CAD build for the part. Positions are in the model's coordinates, mm. A direction names the side the tool comes from. Coordinates: 2 decimals unless noted, no trailing zeros. Write each loop counter-clockwise with the first axis right and the second up, starting at its lowest first coordinate (ties: lowest second). Pieces come first, ordered by that corner, then holes. Notation, with made-up numbers: (27.5, -4.75) - (33.5, -4.75) arc R36 cw to (33.5, 33.25) - close; hole circle Ø2 at (86, -12.5). An arc over 180 degrees is marked (long way). One line per question, with ' | ' between items. Start each with the question number.
1. Band-saw the part on D-D, the plane y = -25. Write the cut outline in (x, z), then the cut area to 3 significant figures.
2. Flat gauge pins, fed straight in: P1, Ø1.5, axis at y = 67, z = 3, coming from the -X side; P2, Ø1, axis at x = 87, y = 21.5, coming from the +Z side. Where does each tip first touch, or does it go through?
3. Band-saw the part on B-B, the plane y = 37. Write the cut outline in (x, z).
4. Probe line 1 (X direction, y = -22, z = 1.15); line 2 (Y direction, x = 71, z = 1.3); line 3 (X direction, y = 14.5, z = 1.85). List the from-to ranges inside material, lowest first.
5. Band-saw the part on C-C, the plane x = 55.5. Write the cut outline in (y, z).
6. Which spindle directions (+Z, -Z, +X, -X, +Y, -Y) get a long thin tool onto all of the face, cutting with end or side? Do faces 1 (the flat face through (113, -11, 2)), 2 (the flat face through (-34.409, 38, 3)), 3 (the flat face through (113, 66.124, 3)), 4 (the flat face through (-29.409, 67, 2)). Say none if no direction does.
7. Band-saw the part on A-A, the plane x = 13. Write the cut outline in (y, z), then the cut area to 3 significant figures.
from build123d import *

# Parameters (mm, degrees)
F0_W     = 160
F0_H     = 110
F1_DEPTH = 2
F2_W     = 155
F2_H     = 5
F3_DEPTH = 3
F4_W     = 0.4
F4_H     = 100.6983700028
F4_H_2   = 0.4
F4_W_2   = 91.7048521668
F4_W_3   = 70
F4_H_3   = 101.3179807599
F4_H_4   = 104.9661831624
F4_H_5   = 97.0501676003
F4_W_4   = 42.9082732886
F5_DEPTH = 0.6
F6_DEPTH = 4
F6_TAPER = -15
F7_R     = 2
F8_W     = 10
F8_H     = 10
F8_W_2   = 47.3290588707
F8_H_2   = 24.0664053708
F8_W_3   = 54.0067385882
F8_H_3   = 33.9830359444
F8_W_4   = 52.8240427375
F8_H_4   = 37.9707552493
F8_W_5   = 50.7075823843
F8_H_5   = 33.7607157417
F9_DEPTH = 25


with BuildPart() as f1:
    # F0 (on Top) → F1 (new body)
    with BuildSketch(Plane.XY):
        with Locations((40.5911064893, 16.1241146261)):
            Rectangle(F0_W, F0_H)
    extrude(amount=F1_DEPTH)

    # F2 (on face) → F3 (join)
    with BuildSketch(Plane.XY.offset(2)):
        Polygon((-34.4088935107, 71.1241146261), (-39.4088935107, 71.1241146261), (-39.4088935107, -38.8758853739), (-34.4088935107, -38.8758853739), (-34.4088935107, 66.1241146261), align=None)
        with Locations((43.0911064893, 68.6241146261)):
            Rectangle(F2_W, F2_H)
    extrude(amount=F3_DEPTH)

    # F4 (on face) → F5 (cut)
    with BuildSketch(Plane.XY.offset(2)):
        with Locations((35.5911064893, 66.6732996275)):
            Rectangle(F4_W, F4_H)
        with Locations((35.5911064893, 16.1241146261)):
            Rectangle(F4_W, F4_H_2)
        with Locations((-10.4613195941, 16.1241146261)):
            Rectangle(F4_W_2, F4_H_2)
        with Locations((70.7911064893, 16.1241146261)):
            Rectangle(F4_W_3, F4_H_2)
        with Locations((35.5911064893, -34.7348757538)):
            Rectangle(F4_W, F4_H_3)
        with Locations((105.9911064893, 16.1241146261)):
            Rectangle(F4_W, F4_H_2)
        with Locations((105.9911064893, 68.8072062073)):
            Rectangle(F4_W, F4_H_4)
        with Locations((105.9911064893, -32.600969174)):
            Rectangle(F4_W, F4_H_5)
        with Locations((127.6452431336, 16.1241146261)):
            Rectangle(F4_W_4, F4_H_2)
    extrude(amount=-F5_DEPTH, mode=Mode.SUBTRACT)

    # F4 (on face) → F6 (cut)
    with BuildSketch(Plane.XY.offset(2)):
        with Locations((35.5911064893, 66.6732996275)):
            Rectangle(F4_W, F4_H)
        with Locations((35.5911064893, 16.1241146261)):
            Rectangle(F4_W, F4_H_2)
        with Locations((-10.4613195941, 16.1241146261)):
            Rectangle(F4_W_2, F4_H_2)
        with Locations((70.7911064893, 16.1241146261)):
            Rectangle(F4_W_3, F4_H_2)
        with Locations((35.5911064893, -34.7348757538)):
            Rectangle(F4_W, F4_H_3)
        with Locations((105.9911064893, 16.1241146261)):
            Rectangle(F4_W, F4_H_2)
        with Locations((105.9911064893, 68.8072062073)):
            Rectangle(F4_W, F4_H_4)
        with Locations((105.9911064893, -32.600969174)):
            Rectangle(F4_W, F4_H_5)
        with Locations((127.6452431336, 16.1241146261)):
            Rectangle(F4_W_4, F4_H_2)
    extrude(amount=F6_DEPTH, taper=F6_TAPER, mode=Mode.SUBTRACT)

    # F7
    f7_edges = [f1.edges().sort_by_distance(p)[0] for p in [
        (-36.908894, 17.127962, 5),
        (-36.908894, 15.120267, 5),
        (34.587259, 68.624115, 5),
        (36.594954, 68.624115, 5),
        (106.994954, 68.624115, 5),
        (104.987259, 68.624115, 5),
    ]]
    fillet(f7_edges, radius=F7_R)

    # F8 (on face) → F9 (cut)
    with BuildSketch(Plane.XY.offset(5)):
        with Locations((-34.4088935107, 66.1241146261)):
            Rectangle(F8_W, F8_H)
        with Locations((-0.7081469521, 41.1217464134)):
            Rectangle(F8_W_2, F8_H_2)
        with Locations((-0.4255371168, -9.683905635)):
            Rectangle(F8_W_3, F8_H_3)
        with Locations((71.6814361513, 41.0866308957)):
            Rectangle(F8_W_4, F8_H_4)
        with Locations((72.29234837, -12.4325060751)):
            Rectangle(F8_W_5, F8_H_5)
    extrude(amount=-F9_DEPTH, mode=Mode.SUBTRACT)


solid = f1.part
Filled in:
1) outline: (-39.41, 0) - (-27.43, 0) - (-27.43, 2) - (-34.41, 2) - (-34.41, 5) - (-39.41, 5) - close; (26.58, 0) - (46.94, 0) - (46.94, 2) - (35.79, 2) - (35.79, 1.4) - (35.39, 1.4) - (35.39, 2) - (26.58, 2) - close; (97.65, 0) - (120.59, 0) - (120.59, 2) - (106.19, 2) - (106.19, 1.4) - (105.79, 1.4) - (105.79, 2) - (97.65, 2) - close | area: 125 mm²
2) P1: stops at x = -29.41 | P2: stops at z = 2
3) outline: (-39.41, 0) - (-24.37, 0) - (-24.37, 2) - (-34.41, 2) - (-34.41, 5) - (-39.41, 5) - close; (22.96, 0) - (45.27, 0) - (45.27, 2) - (35.79, 2) - (35.79, 1.4) - (35.39, 1.4) - (35.39, 2) - (22.96, 2) - close; (98.09, 0) - (120.59, 0) - (120.59, 2) - (106.19, 2) - (106.19, 1.4) - (105.79, 1.4) - (105.79, 2) - (98.09, 2) - close
4) line 1: x = -39.41 to -27.43, 26.58 to 46.94, 97.65 to 120.59 | line 2: y = -38.88 to -29.31, 4.45 to 22.1, 60.07 to 71.12 | line 3: x = -39.41 to 35.39, 35.79 to 105.79, 106.19 to 120.59
5) outline: (-38.88, 0) - (-29.31, 0) - (-29.31, 2) - (-38.88, 2) - close; (4.45, 0) - (22.1, 0) - (22.1, 2) - (16.32, 2) - (16.32, 1.4) - (15.92, 1.4) - (15.92, 2) - (4.45, 2) - close; (60.07, 0) - (71.12, 0) - (71.12, 5) - (66.12, 5) - (66.12, 2) - (60.07, 2) - close
6) face 1: +Z, +X, -Y | face 2: +Z, +X, +Y, -Y | face 3: +Z, +X, -X, -Y | face 4: +Z, -Z, -X, +Y
7) outline: (-38.88, 0) - (-26.68, 0) - (-26.68, 2) - (-38.88, 2) - close; (7.31, 0) - (29.09, 0) - (29.09, 2) - (16.32, 2) - (16.32, 1.4) - (15.92, 1.4) - (15.92, 2) - (7.31, 2) - close; (53.15, 0) - (71.12, 0) - (71.12, 5) - (66.12, 5) - (66.12, 2) - (53.15, 2) - close | area: 119 mm²
